from build123d import *

# Parameters (mm, degrees)
BOSS_EXTRUDE1_DEPTH = 85
FILLET1_R           = 1
CUT_EXTRUDE1_DEPTH  = 86
FILLET2_R           = 0.5
FILLET3_R           = 0.25


with BuildPart() as part:
    # Sketch3 → Boss-Extrude1 (new body)
    with BuildSketch(Plane(origin=(0, 0, 0), x_dir=(1, 0, 0), z_dir=(0, 1, 0))):
        with BuildLine():
            Line((7, 18.5), (7, 19.5))
            ThreePointArc((7, 19.5), (6.646446609, 19.646446609), (6.5, 20))
            Line((6.5, 20), (0, 20))
            Line((0, 20), (0, 13.5))
            ThreePointArc((0, 13.5), (0.353553391, 13.353553391), (0.5, 13))
            Line((0.5, 13), (1.5, 13))
            Line((1.5, 13), (1.5, 16))
            Line((1.5, 16), (3, 16))
            Line((3, 16), (5.5, 13.5))
            Line((5.5, 13.5), (5.5, 10.5))
            Line((5.5, 10.5), (6, 10))
            Line((6, 10), (5.5, 9.5))
            Line((5.5, 9.5), (5.5, 6.5))
            Line((5.5, 6.5), (3, 4))
            Line((3, 4), (1.5, 4))
            Line((1.5, 4), (1.5, 7))
            Line((1.5, 7), (0.5, 7))
            ThreePointArc((0.5, 7), (0.353553391, 6.646446609), (0, 6.5))
            Line((0, 6.5), (0, 0))
            Line((0, 0), (6.5, 0))
            ThreePointArc((6.5, 0), (6.646446609, 0.353553391), (7, 0.5))
            Line((7, 0.5), (7, 1.5))
            Line((7, 1.5), (4, 1.5))
            Line((4, 1.5), (4, 3))
            Line((4, 3), (6.5, 5.5))
            Line((6.5, 5.5), (9.5, 5.5))
            Line((9.5, 5.5), (10, 6))
            Line((10, 6), (10.5, 5.5))
            Line((10.5, 5.5), (13.5, 5.5))
            Line((13.5, 5.5), (16, 3))
            Line((16, 3), (16, 1.5))
            Line((16, 1.5), (13, 1.5))
            Line((13, 1.5), (13, 0.5))
            ThreePointArc((13, 0.5), (13.353553391, 0.353553391), (13.5, 0))
            Line((13.5, 0), (20, 0))
            Line((20, 0), (20, 6.5))
            ThreePointArc((20, 6.5), (19.646446609, 6.646446609), (19.5, 7))
            Line((19.5, 7), (18.5, 7))
            Line((18.5, 7), (18.5, 4))
            Line((18.5, 4), (17, 4))
            Line((17, 4), (14.5, 6.5))
            Line((14.5, 6.5), (14.5, 9.5))
            Line((14.5, 9.5), (14, 10))
            Line((14, 10), (14.5, 10.5))
            Line((14.5, 10.5), (14.5, 13.5))
            Line((14.5, 13.5), (17, 16))
            Line((17, 16), (18.5, 16))
            Line((18.5, 16), (18.5, 13))
            Line((18.5, 13), (19.5, 13))
            ThreePointArc((19.5, 13), (19.646446609, 13.353553391), (20, 13.5))
            Line((20, 13.5), (20, 20))
            Line((20, 20), (13.5, 20))
            ThreePointArc((13.5, 20), (13.353553391, 19.646446609), (13, 19.5))
            Line((13, 19.5), (13, 18.5))
            Line((13, 18.5), (16, 18.5))
            Line((16, 18.5), (16, 17))
            Line((16, 17), (13.5, 14.5))
            Line((13.5, 14.5), (10.5, 14.5))
            Line((10.5, 14.5), (10, 14))
            Line((10, 14), (9.5, 14.5))
            Line((9.5, 14.5), (6.5, 14.5))
            Line((6.5, 14.5), (4, 17))
            Line((4, 17), (4, 18.5))
            Line((4, 18.5), (7, 18.5))
        make_face()
    extrude(amount=BOSS_EXTRUDE1_DEPTH)

    # Fillet1
    fillet1_edges = [part.edges().sort_by_distance(p)[0] for p in [
        (20, 42.5, 0),
        (0, 42.5, 0),
        (0, 42.5, -20),
        (20, 42.5, -20),
    ]]
    fillet(fillet1_edges, radius=FILLET1_R)

    # Sketch4 → Cut-Extrude1 (cut, through all)
    with BuildSketch(Plane(origin=(0, 85, 0), x_dir=(1, 0, 0), z_dir=(0, 1, 0))):
        with BuildLine():
            Line((10, 11), (11.195582496, 12.195582496))
            ThreePointArc((11.195582496, 12.195582496), (10, 12.5), (8.804417504, 12.195582496))
            Line((8.804417504, 12.195582496), (10, 11))
        make_face()
        with BuildLine():
            ThreePointArc((12.195582496, 11.195582496), (11.767766953, 11.767766953), (11.195582496, 12.195582496))
            Line((11.195582496, 12.195582496), (10, 11))
            Line((10, 11), (11, 10))
            Line((11, 10), (12.195582496, 11.195582496))
        make_face()
        with BuildLine():
            Line((9, 10), (10, 11))
            Line((10, 11), (8.804417504, 12.195582496))
            ThreePointArc((8.804417504, 12.195582496), (8.232233047, 11.767766953), (7.804417504, 11.195582496))
            Line((7.804417504, 11.195582496), (9, 10))
        make_face()
        Polygon((11, 10), (10, 11), (9, 10), (10, 9), align=None)
        with BuildLine():
            Line((7.804417504, 8.804417504), (9, 10))
            Line((9, 10), (7.804417504, 11.195582496))
            ThreePointArc((7.804417504, 11.195582496), (7.5, 10), (7.804417504, 8.804417504))
        make_face()
        with BuildLine():
            Line((10, 9), (9, 10))
            Line((9, 10), (7.804417504, 8.804417504))
            ThreePointArc((7.804417504, 8.804417504), (8.232233047, 8.232233047), (8.804417504, 7.804417504))
            Line((8.804417504, 7.804417504), (10, 9))
        make_face()
        with BuildLine():
            Line((11.195582496, 7.804417504), (10, 9))
            Line((10, 9), (8.804417504, 7.804417504))
            ThreePointArc((8.804417504, 7.804417504), (10, 7.5), (11.195582496, 7.804417504))
        make_face()
        with BuildLine():
            Line((12.195582496, 8.804417504), (11, 10))
            Line((11, 10), (10, 9))
            Line((10, 9), (11.195582496, 7.804417504))
            ThreePointArc((11.195582496, 7.804417504), (11.767766953, 8.232233047), (12.195582496, 8.804417504))
        make_face()
        with BuildLine():
            ThreePointArc((12.5, 10), (12.422700584, 10.616864556), (12.195582496, 11.195582496))
            Line((12.195582496, 11.195582496), (11, 10))
            Line((11, 10), (12.195582496, 8.804417504))
            ThreePointArc((12.195582496, 8.804417504), (12.422700584, 9.383135444), (12.5, 10))
        make_face()
        with BuildLine():
            ThreePointArc((8.804417504, 7.804417504), (8.232233047, 8.232233047), (7.804417504, 8.804417504))
            Line((7.804417504, 8.804417504), (7, 8))
            Line((7, 8), (8, 7))
            Line((8, 7), (8.804417504, 7.804417504))
        make_face()
        with BuildLine():
            Line((13, 8), (12.195582496, 8.804417504))
            ThreePointArc((12.195582496, 8.804417504), (11.767766953, 8.232233047), (11.195582496, 7.804417504))
            Line((11.195582496, 7.804417504), (12, 7))
            Line((12, 7), (13, 8))
        make_face()
        with BuildLine():
            Line((13, 12), (12, 13))
            Line((12, 13), (11.195582496, 12.195582496))
            ThreePointArc((11.195582496, 12.195582496), (11.767766953, 11.767766953), (12.195582496, 11.195582496))
            Line((12.195582496, 11.195582496), (13, 12))
        make_face()
        with BuildLine():
            ThreePointArc((7.804417504, 11.195582496), (8.232233047, 11.767766953), (8.804417504, 12.195582496))
            Line((8.804417504, 12.195582496), (8, 13))
            Line((8, 13), (7, 12))
            Line((7, 12), (7.804417504, 11.195582496))
        make_face()
    extrude(amount=-CUT_EXTRUDE1_DEPTH, mode=Mode.SUBTRACT)

    # Fillet2
    fillet2_edges = [part.edges().sort_by_distance(p)[0] for p in [
        (18.5, 42.5, -13),
        (18.5, 42.5, -16),
        (14.5, 42.5, -10.5),
        (14.5, 42.5, -9.5),
        (18.5, 42.5, -4),
        (18.5, 42.5, -7),
        (13, 42.5, -1.5),
        (16, 42.5, -1.5),
        (10.5, 42.5, -5.5),
        (9.5, 42.5, -5.5),
        (4, 42.5, -1.5),
        (7, 42.5, -1.5),
        (1.5, 42.5, -7),
        (1.5, 42.5, -4),
        (5.5, 42.5, -9.5),
        (5.5, 42.5, -10.5),
        (1.5, 42.5, -16),
        (1.5, 42.5, -13),
        (7, 42.5, -18.5),
        (4, 42.5, -18.5),
        (9.5, 42.5, -14.5),
        (10.5, 42.5, -14.5),
        (16, 42.5, -18.5),
        (13, 42.5, -18.5),
    ]]
    fillet(fillet2_edges, radius=FILLET2_R)

    # Fillet3
    fillet3_edges = [part.edges().sort_by_distance(p)[0] for p in [
        (7, 42.5, -12),
        (8, 42.5, -13),
        (12, 42.5, -13),
        (13, 42.5, -12),
        (13, 42.5, -8),
        (12, 42.5, -7),
        (8, 42.5, -7),
        (7, 42.5, -8),
    ]]
    fillet(fillet3_edges, radius=FILLET3_R)


solid = part.part
Read the model definition and answer for the solid it produces. Units are mm, in the model's axes. Coordinates: 2 decimals unless noted, no trailing zeros.
Q1. The mould has two halves that part along Z. Classify faces 1 (the face through (1.5, 42, -5)), 2 (the face through (0, 42, -16)): +Z half, -Z half, draft (parallel to the pull), parting line (faces both ways), or undercut.
Q2. Each of these flat-tipped pins is pushed along its axis until it touches: pin 1 Ø0.8 at (x, y) = (12.5, 45) entering from +Z; pin 2 Ø10 at (x, z) = (8, -3) entering from -Y; pin 3 Ø2 at (x, y) = (8.5, 48.5) entering from -Z; pin 4 Ø1.4 at (y, z) = (32, -7.5) entering from +X. Where does it stop, or does it pass through?
Q3. Consider probe 1 along X at (y, z) = (36, -5); probe 2 along Z at (x, y) = (8, 27); probe 3 along X at (y, z) = (39.5, -13.75). Determine where each line is inside the solid, lowest interval first.
Results below:
1. face 1: undercut
1. face 2: draft
2. pin 1: stops at z = -5.5
2. pin 2: stops at y = 0
2. pin 3: stops at z = -14.5
2. pin 4: stops at x = 19.54
3. probe 1: x = 0 to 1.5, 4 to 6, 14 to 16, 18.5 to 20
3. probe 2: z = -14.5 to -12.9, -7.1 to -5.5
3. probe 3: x = 0 to 1.5, 5.25 to 14.75, 18.5 to 20
